For this review, take the finished solid that the model builds, in its own axes (mm). Coordinates: 2 decimals unless noted, no trailing zeros. Order: outer loops, then holes, each group sorted by start corner. A loop starts at its lowest first (then second) coordinate and runs counter-clockwise, first axis right, second up. Notation, with made-up numbers: (78, 20.5) -> (137, 20.5) arc R12 cw to (137, 28.5) -> close; hole circle Ø3 at (66.25, 13.25). An arc over 180 degrees is marked (long way). Write item = value, one per line. Start each with the question number.
1) Draft analysis for pull direction Z (two halves, no side actions). For faces 1 (the face through (75, 63, 0)), 2 (the face through (75, 127, -26)), 3 (the face through (75.13, 101.75, -26.78)), state which applies: +Z half, -Z half, draft (parallel to the pull), parting line (faces both ways), or undercut.
2) Consider section B-B on y = 19.05. Give the boundary of the cut face in (x, z), and give its area (3 significant figures).
3) Consider section C-C on x = 23. Give the boundary of the cut face in (y, z), and give its area (3 significant figures).
4) Consider section A-A on z = -25.4. Give the boundary of the cut face in (x, y).
5) Wall thickness on probe 1 along Y at (x, z) = (37, -25); probe 2 along Y at (x, z) = (44.5, -26.5); probe 3 along Z at (x, y) = (43, 19): over which ranges is each line inside the solid? List them lowest first. Write a range as [from, to].
from build123d import *

# Parameters (mm, degrees)
SKETCH1_W           = 152.4
SKETCH1_H           = 50.8
BOSS_EXTRUDE1_DEPTH = 127
SKETCH3_R           = 6.35
CUT_EXTRUDE1_DEPTH  = 153.4


with BuildPart() as part:
    # Sketch1 → Boss-Extrude1 (new body)
    with BuildSketch(Plane(origin=(0, 0, 0), x_dir=(1, 0, 0), z_dir=(0, 1, 0))):
        with Locations((76.2, 25.4)):
            Rectangle(SKETCH1_W, SKETCH1_H)
    extrude(amount=BOSS_EXTRUDE1_DEPTH)

    # Sketch3 → Cut-Extrude1 (cut, through all)
    with BuildSketch(Plane.ZY):
        with Locations((-25.4, 19.05)):
            Circle(SKETCH3_R)
        with Locations((-25.4, 107.95)):
            Circle(SKETCH3_R)
    extrude(amount=-CUT_EXTRUDE1_DEPTH, mode=Mode.SUBTRACT)


solid = part.part
Answer sheet:
q1.face_1 = +Z half
q1.face_2 = draft
q1.face_3 = undercut
q2.outline = (0, -50.8) -> (152.4, -50.8) -> (152.4, -31.75) -> (0, -31.75) -> close; (0, -19.05) -> (152.4, -19.05) -> (152.4, 0) -> (0, 0) -> close
q2.area = 5,810 mm2
q3.outline = (0, -50.8) -> (127, -50.8) -> (127, 0) -> (0, 0) -> close; hole circle Ø12.7 at (19.05, -25.4); hole circle Ø12.7 at (107.95, -25.4)
q3.area = 6,200 mm2
q4.outline = (0, 0) -> (152.4, 0) -> (152.4, 12.7) -> (0, 12.7) -> close; (0, 25.4) -> (152.4, 25.4) -> (152.4, 101.6) -> (0, 101.6) -> close; (0, 114.3) -> (152.4, 114.3) -> (152.4, 127) -> (0, 127) -> close
q5.probe_1 = [0, 12.71], [25.39, 101.61], [114.29, 127]
q5.probe_2 = [0, 12.8], [25.3, 101.7], [114.2, 127]
q5.probe_3 = [-50.8, -31.75], [-19.05, 0]
